from build123d import *

# Parameters (mm, degrees)
SKETCH107_W     = 92.613678
SKETCH107_H     = 150
SKETCH107_R     = 1.7
PAD044_DEPTH    = 4
SKETCH106_R     = 42.5
PAD043_DEPTH    = 13.5
SKETCH105_R     = 35.15
SKETCH105_R_2   = 31.5
PAD042_DEPTH    = 12
SKETCH130_R     = 31.5
POCKET023_DEPTH = 20


with BuildPart() as part:
    # Sketch107 → Pad044 (new body)
    with BuildSketch(Plane.XY):
        with Locations((0, -17.3981255757)):
            Rectangle(SKETCH107_W, SKETCH107_H)
        with Locations((-27.6317588753, 49.5634491508)):
            Circle(SKETCH107_R, mode=Mode.SUBTRACT)
        with Locations((27.6317588753, 49.5634491508)):
            Circle(SKETCH107_R, mode=Mode.SUBTRACT)
        with Locations((27.6317588753, -85.4365508492)):
            Circle(SKETCH107_R, mode=Mode.SUBTRACT)
        with Locations((-27.6317588753, -85.4365508492)):
            Circle(SKETCH107_R, mode=Mode.SUBTRACT)
        with BuildLine():
            ThreePointArc((-23.0708364387, -46.4607558182), (-39.1290583868, -62.5189777662), (-23.0708364387, -78.5771997143))
            Line((-23.0708364387, -78.5771997143), (23.317797, -78.5771997143))
            ThreePointArc((23.317797, -78.5771997143), (39.3760189481, -62.5189777662), (23.317797, -46.4607558182))
            Line((-23.0708364387, -46.4607558182), (23.317797, -46.4607558182))
        make_face(mode=Mode.SUBTRACT)
    extrude(amount=PAD044_DEPTH)

    # Sketch106 (on Face13 of Pad044) → Pad043 (join)
    with BuildSketch(Plane(origin=(0, 0, 0), x_dir=(1, 0, 0), z_dir=(0, 0, -1))):
        Circle(SKETCH106_R)
    extrude(amount=PAD043_DEPTH)

    # Sketch105 (on Face16 of Pad043) → Pad042 (join)
    with BuildSketch(Plane(origin=(0, 0, -13.5), x_dir=(1, 0, 0), z_dir=(0, 0, -1))):
        Circle(SKETCH105_R)
        Circle(SKETCH105_R_2, mode=Mode.SUBTRACT)
    extrude(amount=PAD042_DEPTH)

    # Sketch130 (on Face20 of Pad042) → Pocket023 (cut)
    with BuildSketch(Plane(origin=(0, 0, -13.5), x_dir=(1, 0, 0), z_dir=(0, 0, -1))):
        Circle(SKETCH130_R)
    extrude(amount=-POCKET023_DEPTH, mode=Mode.SUBTRACT)


with BuildPart() as part_1:
    # Body012 placement: moved
    add(part.part.moved(Location((-18.5, 10, 19))))


solid = part_1.part
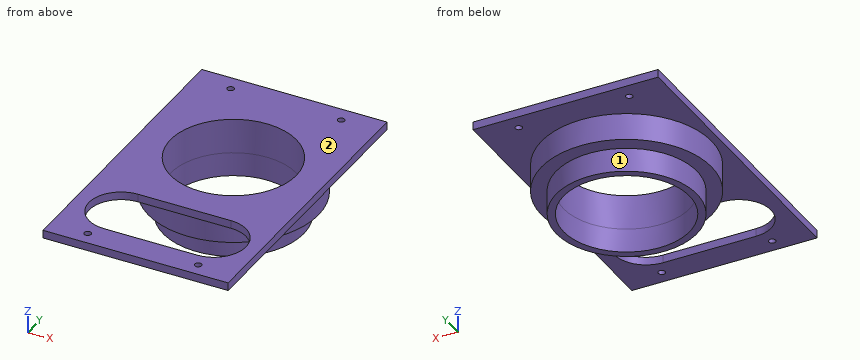
Can you work these out from the model? Positions are in its coordinate system, mm. Face numbers are marked on the shaded views. A direction names the side the tool comes from. Coordinates: 2 decimals unless noted, no trailing zeros. Write each loop counter-clockwise with the first axis right and the second up, starting at its lowest first coordinate (ties: lowest second). Pieces come first, ordered by that corner, then holes. Notation, with made-up numbers: (19, 69) -> (28, 69) arc R17 cw to (28, 79) -> close; hole circle Ø5 at (-1, 39). An arc over 180 degrees is marked (long way). Write each question's results on one line, items separated by ' | '. Start each with the question number.
Q1. Imagine slicing it at C-C (z = 8.5). Write out the boundary of the cut face in (x, y).
Q2. On a 3-axis mill with a long thin cutter (end or side, diameter ignored), from which of +Z, -Z, +X, -X, +Y, -Y can I reach the whole of each face in a straight line? I mean the marked faces 1 and 2. Say none if no direction works.
Q3. Imagine slicing it at B-B (x = -18.5). Write out the boundary of the cut face in (y, z).
Q4. I'm going to push flat-ended pins straight in: pin 1 (2.5 mm diameter, centred on x = 9.13, y = -75.44, fed in from +Z); pin 2 (5 mm diameter, centred on x = -36, z = 12, fed in from +Y); pin 3 (12 mm diameter, centred on y = 13.5, z = 5.5, fed in from +X); pin 4 (8 mm diameter, centred on x = -46.5, z = 0.5, fed in from +Y). Where does each tip first touch, or does it pass through?
Q5. Imagine slicing it at D-D (y = -38). Write out the boundary of the cut face in (x, z), then the cut area to 3 significant figures.
Q6. If I drill on probe 1 along Y at (x, z) = (-18.5, 18); probe 2 along Y at (x, z) = (4, 19.75); probe 3 along X at (y, z) = (10, 0), over which ranges is the centre line in solid material (lowest first)?
Q7. Imagine slicing it at A-A (y = 10). Write out the boundary of the cut face in (x, z).
Taken from the geometry:
1) outline: circle Ø85 at (-18.5, 10); hole circle Ø63 at (-18.5, 10)
2) face 1: -Z | face 2: +Z, +X, -X, +Y, -Y
3) outline: (-82.4, 19) -> (-68.58, 19) -> (-68.58, 23) -> (-82.4, 23) -> close; (-36.46, 19) -> (-32.5, 19) -> (-32.5, 5.5) -> (-25.15, 5.5) -> (-25.15, -6.5) -> (-21.5, -6.5) -> (-21.5, 23) -> (-36.46, 23) -> close; (41.5, -6.5) -> (45.15, -6.5) -> (45.15, 5.5) -> (52.5, 5.5) -> (52.5, 19) -> (67.6, 19) -> (67.6, 23) -> (41.5, 23) -> close
4) pin 1: passes through | pin 2: stops at y = 49.76 | pin 3: stops at x = 24 | pin 4: stops at y = 35.68
5) outline: (-64.81, 19) -> (-48.43, 19) -> (-48.43, 23) -> (-64.81, 23) -> close; (11.68, 19) -> (27.81, 19) -> (27.81, 23) -> (11.68, 23) -> close | area: 130 mm^2
6) probe 1: y = -32.5 to -21.5, 41.5 to 52.5 | probe 2: y = -82.4 to -68.58, -36.46 to -12.05, 32.05 to 67.6 | probe 3: x = -53.65 to -50, 13 to 16.65
7) outline: (-64.81, 19) -> (-61, 19) -> (-61, 5.5) -> (-53.65, 5.5) -> (-53.65, -6.5) -> (-50, -6.5) -> (-50, 23) -> (-64.81, 23) -> close; (13, -6.5) -> (16.65, -6.5) -> (16.65, 5.5) -> (24, 5.5) -> (24, 19) -> (27.81, 19) -> (27.81, 23) -> (13, 23) -> close
